For this review, take the finished solid that the model builds, in its own axes (mm). A direction names the side the tool comes from. Round coordinates to 2 decimals unless told otherwise and drop trailing zeros. Order: outer loops, then holes, each group sorted by start corner. A loop starts at its lowest first (then second) coordinate and runs counter-clockwise, first axis right, second up. Notation, with made-up numbers: M 0,40 L 37,40 A21 ccw 37,74 Z; hole C 0,-30.75 d4. An arc over 180 degrees is marked long. Answer in a Markdown table with one row per item. Add a question column.
```python
from build123d import *

# Parameters (mm, degrees)
SKETCH3_W            = 50.8
SKETCH3_H            = 50.8
BOSS_EXTRUDE1_DEPTH  = 88.9
SKETCH4_W            = 50.8
SKETCH4_H            = 50.8
BOSS_EXTRUDE2_DEPTH  = 88.9
SKETCH5_W            = 50.8
SKETCH5_H            = 50.8
BOSS_EXTRUDE3_DEPTH  = 88.9
FILLET1_R            = 0.1
FILLET2_R            = 0.1
FILLET3_R            = 0.1
SKETCH6_W            = 50.8
SKETCH6_H            = 50.8
BOSS_EXTRUDE4_DEPTH  = 88.9
FILLET4_R            = 0.1
SKETCH8_W            = 50.8
SKETCH8_H            = 50.8
BOSS_EXTRUDE5_DEPTH  = 88.9
SKETCH9_W            = 50.8
SKETCH9_H            = 50.8
BOSS_EXTRUDE6_DEPTH  = 88.9
FILLET5_R            = 2.54
FILLET6_R            = 2.54
SKETCH10_W           = 1143
SKETCH10_H           = 635
BOSS_EXTRUDE7_DEPTH  = 1117.6
SKETCH11_W           = 495.3
SKETCH11_H           = 253.909609279
CUT_EXTRUDE1_DEPTH   = 558.8
FILLET7_R            = 2.54
LPATTERN1_COUNT      = 3
LPATTERN1_PITCH      = 355.6
LPATTERN1_COUNT_DIR2 = 2
LPATTERN1_PITCH_DIR2 = 546.1
SKETCH13_R           = 31.75
CUT_EXTRUDE2_DEPTH   = 970.026


with BuildPart() as part:
    # Sketch3 → Boss-Extrude1 (new body)
    with BuildSketch(Plane(origin=(0, 0, 0), x_dir=(1, 0, 0), z_dir=(0, 1, 0))):
        with Locations((546.1, 292.1)):
            Rectangle(SKETCH3_W, SKETCH3_H)
    extrude(amount=BOSS_EXTRUDE1_DEPTH)

    # Fillet2
    fillet2_edges = [part.edges().sort_by_distance(p)[0] for p in [
        (520.7, 44.45, -317.5),
        (571.5, 44.45, -317.5),
        (571.5, 44.45, -266.7),
        (520.7, 44.45, -266.7),
    ]]
    fillet(fillet2_edges, radius=FILLET2_R)



with BuildPart() as body_2:
    # Sketch4 → Boss-Extrude2 (new body)
    with BuildSketch(Plane(origin=(0, 0, 0), x_dir=(1, 0, 0), z_dir=(0, 1, 0))):
        with Locations((546.1, -292.1)):
            Rectangle(SKETCH4_W, SKETCH4_H)
    extrude(amount=BOSS_EXTRUDE2_DEPTH)

    # Fillet1
    fillet1_edges = [body_2.edges().sort_by_distance(p)[0] for p in [
        (520.7, 44.45, 266.7),
        (571.5, 44.45, 266.7),
        (571.5, 44.45, 317.5),
        (520.7, 44.45, 317.5),
    ]]
    fillet(fillet1_edges, radius=FILLET1_R)


with BuildPart() as body_3:
    # Sketch5 → Boss-Extrude3 (new body)
    with BuildSketch(Plane(origin=(0, 0, 0), x_dir=(1, 0, 0), z_dir=(0, 1, 0))):
        with Locations((-546.1, 292.1)):
            Rectangle(SKETCH5_W, SKETCH5_H)
    extrude(amount=BOSS_EXTRUDE3_DEPTH)

    # Fillet3
    fillet3_edges = [body_3.edges().sort_by_distance(p)[0] for p in [
        (-520.7, 44.45, -266.7),
        (-571.5, 44.45, -266.7),
        (-571.5, 44.45, -317.5),
        (-520.7, 44.45, -317.5),
    ]]
    fillet(fillet3_edges, radius=FILLET3_R)


with BuildPart() as body_4:
    # Sketch6 → Boss-Extrude4 (new body)
    with BuildSketch(Plane(origin=(0, 0, 0), x_dir=(1, 0, 0), z_dir=(0, 1, 0))):
        with Locations((-546.1, -292.1)):
            Rectangle(SKETCH6_W, SKETCH6_H)
    extrude(amount=BOSS_EXTRUDE4_DEPTH)

    # Fillet4
    fillet4_edges = [body_4.edges().sort_by_distance(p)[0] for p in [
        (-520.7, 44.45, 317.5),
        (-571.5, 44.45, 317.5),
        (-571.5, 44.45, 266.7),
        (-520.7, 44.45, 266.7),
    ]]
    fillet(fillet4_edges, radius=FILLET4_R)


with BuildPart() as body_5:
    # Sketch8 → Boss-Extrude5 (new body)
    with BuildSketch(Plane(origin=(0, 0, 0), x_dir=(1, 0, 0), z_dir=(0, 1, 0))):
        with Locations((0, 292.1)):
            Rectangle(SKETCH8_W, SKETCH8_H)
    extrude(amount=BOSS_EXTRUDE5_DEPTH)

    # Fillet6
    fillet6_edges = [body_5.edges().sort_by_distance(p)[0] for p in [
        (25.4, 44.45, -266.7),
        (-25.4, 44.45, -266.7),
        (-25.4, 44.45, -317.5),
        (25.4, 44.45, -317.5),
    ]]
    fillet(fillet6_edges, radius=FILLET6_R)


with BuildPart() as body_6:
    # Sketch9 → Boss-Extrude6 (new body)
    with BuildSketch(Plane(origin=(0, 0, 0), x_dir=(1, 0, 0), z_dir=(0, 1, 0))):
        with Locations((0, -292.1)):
            Rectangle(SKETCH9_W, SKETCH9_H)
    extrude(amount=BOSS_EXTRUDE6_DEPTH)

    # Fillet5
    fillet5_edges = [body_6.edges().sort_by_distance(p)[0] for p in [
        (25.4, 44.45, 317.5),
        (-25.4, 44.45, 317.5),
        (-25.4, 44.45, 266.7),
        (25.4, 44.45, 266.7),
    ]]
    fillet(fillet5_edges, radius=FILLET5_R)


with BuildPart() as part_1:
    add(part.part)

    add(body_2.part)  # Boss-Extrude7 merges body 2

    add(body_3.part)  # Boss-Extrude7 merges body 3

    add(body_4.part)  # Boss-Extrude7 merges body 4

    add(body_5.part)  # Boss-Extrude7 merges body 5

    add(body_6.part)  # Boss-Extrude7 merges body 6
    # Sketch10 → Boss-Extrude7 (add)
    with BuildSketch(Plane(origin=(0, 88.9, 0), x_dir=(1, 0, 0), z_dir=(0, 1, 0))):
        Rectangle(SKETCH10_W, SKETCH10_H)
    extrude(amount=BOSS_EXTRUDE7_DEPTH)

    # Sketch11 → Cut-Extrude1 (cut)
    with BuildSketch(Plane.XY.offset(317.5)):
        with Locations((-273.05, 266.65480464)):
            Rectangle(SKETCH11_W, SKETCH11_H)
    cut_extrude1 = extrude(amount=-CUT_EXTRUDE1_DEPTH, mode=Mode.SUBTRACT)

    # Fillet7
    fillet7_edges = [part_1.edges().sort_by_distance(p)[0] for p in [
        (-571.5, 1206.5, 0),
        (0, 1206.5, 317.5),
        (0, 1206.5, -317.5),
        (571.5, 1206.5, 0),
        (571.5, 647.7, -317.5),
        (571.5, 647.7, 317.5),
        (-571.5, 647.7, 317.5),
    ]]
    fillet(fillet7_edges, radius=FILLET7_R)

    # LPattern1: Cut-Extrude1 3 × 2
    with Locations(*[(j * LPATTERN1_PITCH_DIR2, i * LPATTERN1_PITCH, 0) for i in range(LPATTERN1_COUNT) for j in range(LPATTERN1_COUNT_DIR2) if (i, j) != (0, 0)]):
        add(cut_extrude1, mode=Mode.SUBTRACT)

    # Sketch13 → Cut-Extrude2 (cut)
    with BuildSketch(Plane(origin=(0, 1206.5, 0), x_dir=(1, 0, 0), z_dir=(0, 1, 0))):
        with Locations(Location((492.76, 241.3, 0), (0, 0, 270))):
            Circle(SKETCH13_R)
    extrude(amount=-CUT_EXTRUDE2_DEPTH, mode=Mode.SUBTRACT)


solid = part_1.part
```
1. Clearance check with flat-ended pins moving along their axes: pin 1 Ø4 at (x, z) = (173, -20.5) entering from -Y; pin 2 Ø2 at (x, y) = (-95.5, 682) entering from +Z. State where each tip first meets the part, or that it passes through.
2. Consider section B-B on x = 492.76. Write out the cut boundary in (y, z).
3. The part is to be moulded in two halves that separate along X. For faces 1 (the flat face through (571.5, 594, 4)), 2 (the flat face through (0, 0, -292)), 3 (the flat face through (-520.7, 44, 292)), say which applies: pulls with the +X half, pulls with the -X half, needs draft (parallel to the pull), parting line crosses it, or undercut.
4. For faces 4 (the flat face through (25.4, 44, -292)), 5 (the flat face through (-277, 393.61, 42)), 6 (the flat face through (0, 0, 292)), 7 (the flat face through (-9, 594, -317.5)), 8 (the flat face through (546, 44, -266.7)), list the 3-axis set-ups (+Z, -Z, +X, -X, +Y, -Y) from which the entire face can be reached by the end or side of a thin tool; tool diameter is ignored.
5. Consider section C-C on y = 908.5. Write out the cut boundary in (x, z).
6. Consider section A-A on z = 4.5. State how many separate pieces and enclosed holes the cut face has, plus the area to 3 significant figures.
7. Consider section D-D on x = 284. Write out the cut boundary in (y, z).
8. To check wall thickness, follow probe 1 along Y at (x, z) = (-451.5, 234.5); probe 2 along X at (y, z) = (646, 69.5); probe 3 along X at (y, z) = (511, -241). State the ranges of each line that lie inside material, in increasing order. Write a range as [from, to].
Solved:
| question | item | result |
|---|---|---|
| 1 | pin 1 | stops at y = 88.9 |
| 1 | pin 2 | stops at z = -241.3 |
| 2 | outline | M 88.9,-317.5 L 1203.96,-317.5 A2.54 ccw 1206.5,-314.96 L 1206.5,-273.05 L 236.47,-273.05 L 236.47,-241.3 L 139.7,-241.3 L 139.7,317.5 L 88.9,317.5 Z; M 393.61,-209.55 L 495.3,-209.55 L 495.3,317.5 L 393.61,317.5 Z; M 749.21,-209.55 L 850.9,-209.55 L 850.9,317.5 L 749.21,317.5 Z; M 1104.81,-209.55 L 1206.5,-209.55 L 1206.5,314.96 A2.54 ccw 1203.96,317.5 L 1104.81,317.5 Z |
| 3 | face 1 | pulls with the +X half |
| 3 | face 2 | needs draft |
| 3 | face 3 | undercut |
| 4 | face 4 | +Z, -Z, -Y |
| 4 | face 5 | +Z |
| 4 | face 6 | +Z, -Z, +X, -X, -Y |
| 4 | face 7 | -Z, +X, -X, +Y, -Y |
| 4 | face 8 | +X, -X, -Y |
| 5 | outline | M -571.5,-317.5 L 568.96,-317.5 A2.54 ccw 571.5,-314.96 L 571.5,314.96 A2.54 ccw 568.96,317.5 L 520.7,317.5 L 520.7,-226.22 A31.75 cw long 461.01,-241.3 L 25.4,-241.3 L 25.4,317.5 L -25.4,317.5 L -25.4,-241.3 L -520.7,-241.3 L -520.7,317.5 L -568.96,317.5 A2.54 ccw -571.5,314.96 Z |
| 6 | separate pieces | 1 |
| 6 | enclosed holes | 6 |
| 6 | area | 523,000 mm^2 |
| 7 | outline | M 88.9,-317.5 L 1203.96,-317.5 A2.54 ccw 1206.5,-314.96 L 1206.5,314.96 A2.54 ccw 1203.96,317.5 L 1104.81,317.5 L 1104.81,-241.3 L 850.9,-241.3 L 850.9,317.5 L 749.21,317.5 L 749.21,-241.3 L 495.3,-241.3 L 495.3,317.5 L 393.61,317.5 L 393.61,-241.3 L 139.7,-241.3 L 139.7,317.5 L 88.9,317.5 Z |
| 8 | probe 1 | y = [88.9, 139.7], [393.61, 495.3], [749.21, 850.9], [1104.81, 1206.5] |
| 8 | probe 2 | x = [-571.5, -520.7], [-25.4, 25.4], [520.7, 571.5] |
| 8 | probe 3 | x = [-571.5, -520.7], [-25.4, 25.4], [524.51, 571.5] |
